```python
from build123d import *

# Parameters (mm, degrees)
F1_DEPTH       = 4
F3_DEPTH       = 25
F4_R           = 22.5
F4_R_2         = 12.6
F5_DEPTH       = 30
F6_R           = 12.6
F7_DEPTH       = 25
F9_DEPTH       = 20
F9_DEPTH_BACK  = 20
F11_DEPTH      = 20
F11_DEPTH_BACK = 20
F13_DEPTH      = 60.001
F13_DEPTH_BACK = 85.001
F14_R          = 2.6
F15_DEPTH      = 82.066510674
F15_DEPTH_BACK = 82.066510674
F16_R          = 27.25
F16_R_2        = 24.75
F17_DEPTH      = 3


with BuildPart() as f1:
    # F0 (on Top) → F1 (new body)
    with BuildSketch(Plane.XY):
        with BuildLine():
            ThreePointArc((82.1416340365, -21.8575377801), (84.2823792174, -11.0218216937), (85, 0))
            ThreePointArc((85, 0), (84.2823792174, 11.0218216937), (82.1416340365, 21.8575377801))
            Line((82.1416340365, 21.8575377801), (-22.1416340365, 82.065510674))
            ThreePointArc((-22.1416340365, 82.065510674), (-42.5, 73.6121593217), (-60, 60.207972894))
            Line((-60, 60.207972894), (-60, -60.207972894))
            ThreePointArc((-60, -60.207972894), (-42.5, -73.6121593217), (-22.1416340365, -82.065510674))
            Line((-22.1416340365, -82.065510674), (82.1416340365, -21.8575377801))
        make_face()
    extrude(amount=F1_DEPTH)

    # F2 (on face) → F3 (cut)
    with BuildSketch(Plane.XY.offset(4)):
        with BuildLine():
            ThreePointArc((71.454527972, -2.5495945353), (71.4886310891, -1.275), (71.5, 0))
            ThreePointArc((71.5, 0), (71.4886310891, 1.275), (71.454527972, 2.5495945353))
            ThreePointArc((71.454527972, 2.5495945353), (68.95, 0), (71.454527972, -2.5495945353))
        make_face()
        with BuildLine():
            ThreePointArc((71.454527972, 2.5495945353), (71.4886310891, 1.275), (71.5, 0))
            ThreePointArc((71.5, 0), (71.4886310891, -1.275), (71.454527972, -2.5495945353))
            ThreePointArc((71.454527972, -2.5495945353), (73.2869731851, -1.8191280427), (74.05, 0))
            ThreePointArc((74.05, 0), (73.2869731851, 1.8191280427), (71.454527972, 2.5495945353))
        make_face()
        with BuildLine():
            ThreePointArc((-37.935277623, -60.6066391715), (-37.025, -64.1291811502), (-33.5192503491, -63.1562337069))
            ThreePointArc((-33.5192503491, -63.1562337069), (-35.75, -61.9208163706), (-37.935277623, -60.6066391715))
        make_face()
        with BuildLine():
            ThreePointArc((-37.935277623, -60.6066391715), (-35.75, -61.9208163706), (-33.5192503491, -63.1562337069))
            ThreePointArc((-33.5192503491, -63.1562337069), (-33.2811023097, -62.5588165234), (-33.2, -61.9208163706))
            ThreePointArc((-33.2, -61.9208163706), (-35.0680754949, -59.4636881751), (-37.935277623, -60.6066391715))
        make_face()
        with BuildLine():
            ThreePointArc((-37.935277623, 60.6066391715), (-35.75, 61.9208163706), (-33.5192503491, 63.1562337069))
            ThreePointArc((-33.5192503491, 63.1562337069), (-37.025, 64.1291811502), (-37.935277623, 60.6066391715))
        make_face()
        with BuildLine():
            ThreePointArc((-33.2, 61.9208163706), (-33.2811023097, 62.5588165234), (-33.5192503491, 63.1562337069))
            ThreePointArc((-33.5192503491, 63.1562337069), (-35.75, 61.9208163706), (-37.935277623, 60.6066391715))
            ThreePointArc((-37.935277623, 60.6066391715), (-35.0680754949, 59.4636881751), (-33.2, 61.9208163706))
        make_face()
    extrude(amount=-F3_DEPTH, mode=Mode.SUBTRACT)

    # F4 (on face) → F5 (join)
    with BuildSketch(Plane.XY.offset(4)):
        Circle(F4_R)
        Circle(F4_R_2, mode=Mode.SUBTRACT)
    extrude(amount=F5_DEPTH)

    # F6 (on face) → F7 (cut)
    with BuildSketch(Plane.XY.offset(4)):
        Circle(F6_R)
    extrude(amount=-F7_DEPTH, mode=Mode.SUBTRACT)

    # F8 (on Right) → F9 (cut, two sides)
    with BuildSketch(Plane.YZ) as f9_sk:
        Polygon((-2.3094010768, 11), (2.3094010768, 11), (4.6188021535, 15), (2.3094010768, 19), (-2.3094010768, 19), (-4.6188021535, 15), align=None)
    extrude(amount=F9_DEPTH, mode=Mode.SUBTRACT)
    extrude(f9_sk.sketch, amount=-F9_DEPTH_BACK, mode=Mode.SUBTRACT)

    # F10 (on Front) → F11 (cut, two sides)
    with BuildSketch(Plane.XZ) as f11_sk:
        Polygon((-2.3094010768, 11), (2.3094010768, 11), (4.6188021535, 15), (2.3094010768, 19), (-2.3094010768, 19), (-4.6188021535, 15), align=None)
    extrude(amount=F11_DEPTH, mode=Mode.SUBTRACT)
    extrude(f11_sk.sketch, amount=-F11_DEPTH_BACK, mode=Mode.SUBTRACT)

    # F12 (on Right) → F13 (cut, two sides)
    with BuildSketch(Plane.YZ) as f13_sk:
        with BuildLine():
            ThreePointArc((0, 17.6), (-2.6, 15), (0, 12.4))
            Line((0, 12.4), (0, 17.6))
        make_face()
        with BuildLine():
            Line((0, 17.6), (0, 12.4))
            ThreePointArc((0, 12.4), (1.8384776311, 13.1615223689), (2.6, 15))
            ThreePointArc((2.6, 15), (1.8384776311, 16.8384776311), (0, 17.6))
        make_face()
    extrude(amount=-F13_DEPTH, mode=Mode.SUBTRACT)
    extrude(f13_sk.sketch, amount=F13_DEPTH_BACK, mode=Mode.SUBTRACT)

    # F14 (on Front) → F15 (cut, two sides)
    with BuildSketch(Plane.XZ) as f15_sk:
        with Locations((0, 15)):
            Circle(F14_R)
    extrude(amount=F15_DEPTH, mode=Mode.SUBTRACT)
    extrude(f15_sk.sketch, amount=-F15_DEPTH_BACK, mode=Mode.SUBTRACT)

    # F16 (on face) → F17 (join)
    with BuildSketch(Plane.XY.offset(4)):
        Circle(F16_R)
        Circle(F16_R_2, mode=Mode.SUBTRACT)
    extrude(amount=F17_DEPTH)


solid = f1.part
```
Source: CAD feature listing. Evaluate the final solid. Frame: model axes, mm. A direction names the side the tool comes from. Give positions to 0.01 mm unless a question says otherwise; leave off trailing zeros. Loops run counter-clockwise (first coordinate to the right, second up) from the corner with the lowest first, then second, coordinate; pieces in that order, holes last. Notation, with made-up numbers: (87.25, -8.5) -> (141.25, -8.5) arc R25 cw to (141.25, 22.5) -> close; hole circle Ø8 at (9.5, 35). An arc over 180 degrees is marked (long way). Use a Markdown table: item, result. Add a question column.
(1) Ray query, line 1 (Y direction, x = 0, z = 6.25); line 2 (Z direction, x = 0, y = 21.95); line 3 (Y direction, x = 14.5, z = 5). Return the intervals inside material, ascending.
(2) Section query C-C (z = 28.5). Output: boundary loops of the cut face in (x, y).
(3) Section query A-A (x = -35.75). Output: boundary loops of the cut face in (y, z), then the cut area to 3 significant figures.
(4) Section query B-B (y = -6.5). Output: boundary loops of the cut face in (x, z), then the cut area to 3 significant figures.
(5) First-contact query: pin 1 Ø2 at (x, z) = (20.5, 9) entering from -Y (3 decimals); pin 2 Ø12 at (x, y) = (16, -34) entering from +Z; pin 3 Ø7 at (x, z) = (0, 15) entering from -Y. Flat tips, straight axial feed; report the tip coordinate or a pass-through.
(6) Section query D-D (x = 9.5). Output: boundary loops of the cut face in (y, z).
(7) Pull-direction query (Y, two-part tool) for faces 4 (the face through (10, -10, 34)), 5 (the face through (30.73, 51.54, 1.97)), 6 (the face through (-3.48, 15.8, 13.03)); classes: +Y half, -Y half, draft (parallel to the pull), parting line (faces both ways), or undercut.
(8) Access query for faces 1 (the face through (-3.22, 24.54, 5.48)), 2 (the face through (-15.804, 3.448, 12.972)), 3 (the face through (-5, -17, 0)). Directions: +Z, -Z, +X, -X, +Y, -Y. A direction counts if a zero-diameter tool reaches every point of the face in a straight line with its end or side. Return the directions, or none.
Checked values:
| question | item | result |
|---|---|---|
| 1 | line 1 | -27.25 to -24.75, -22.5 to -12.6, 12.6 to 22.5, 24.75 to 27.25 |
| 1 | line 2 | 0 to 12.4, 17.6 to 34 |
| 1 | line 3 | -23.07 to -20.06, -17.2 to 17.2, 20.06 to 23.07 |
| 2 | outline | circle Ø45 at (0, 0); hole circle Ø25.2 at (0, 0) |
| 3 | outline | (-77.12, 0) -> (-64.47, 0) -> (-64.47, 4) -> (-77.12, 4) -> close; (-59.37, 0) -> (59.37, 0) -> (59.37, 4) -> (-59.37, 4) -> close; (64.47, 0) -> (77.12, 0) -> (77.12, 4) -> (64.47, 4) -> close |
| 3 | area | 576 mm^2 |
| 4 | outline | (-60, 0) -> (-10.79, 0) -> (-10.79, 34) -> (-21.54, 34) -> (-21.54, 4) -> (-23.88, 4) -> (-23.88, 7) -> (-26.46, 7) -> (-26.46, 4) -> (-60, 4) -> close; (10.79, 0) -> (84.75, 0) -> (84.75, 4) -> (26.46, 4) -> (26.46, 7) -> (23.88, 7) -> (23.88, 4) -> (21.54, 4) -> (21.54, 34) -> (10.79, 34) -> close |
| 4 | area | 1,150 mm^2 |
| 5 | pin 1 | y = -11.225 |
| 5 | pin 2 | z = 4 |
| 5 | pin 3 | y = -22.5 |
| 6 | outline | (-63.8, 0) -> (-8.28, 0) -> (-8.28, 34) -> (-20.4, 34) -> (-20.4, 4) -> (-22.85, 4) -> (-22.85, 7) -> (-25.54, 7) -> (-25.54, 4) -> (-63.8, 4) -> close; (8.28, 0) -> (63.8, 0) -> (63.8, 4) -> (25.54, 4) -> (25.54, 7) -> (22.85, 7) -> (22.85, 4) -> (20.4, 4) -> (20.4, 34) -> (8.28, 34) -> close |
| 7 | face 4 | draft |
| 7 | face 5 | +Y half |
| 7 | face 6 | undercut |
| 8 | face 1 | +Z |
| 8 | face 2 | none |
| 8 | face 3 | -Z, +X, -X, +Y, -Y |
